Could you check a few things on this model? Use its own coordinates, in mm. Round coordinates to 2 decimals unless told otherwise and drop trailing zeros. Write each loop counter-clockwise with the first axis right and the second up, starting at its lowest first coordinate (ties: lowest second). Pieces come first, ordered by that corner, then holes. Notation, with made-up numbers: (11.25, 87) -> (31.25, 87) arc R21 cw to (31.25, 97) -> close; hole circle Ø5 at (-23, -14.75). An arc over 180 degrees is marked (long way). Return JSON: item names as keys, results as strings.
from build123d import *

# Parameters (mm, degrees)
SKETCH1_R           = 36.1315
SKETCH1_R_2         = 27.2415
BOSS_EXTRUDE1_DEPTH = 25.4
CUT_EXTRUDE1_START  = -8.908075
SKETCH2_R           = 0.9921875
CUT_EXTRUDE1_DEPTH  = 8.908075
CIRPATTERN1_COUNT   = 4


with BuildPart() as part:
    # Sketch1 → Boss-Extrude1 (new body)
    with BuildSketch(Plane(origin=(0, 0, 0), x_dir=(1, 0, 0), z_dir=(0, 1, 0))):
        Circle(SKETCH1_R)
        Circle(SKETCH1_R_2, mode=Mode.SUBTRACT)
    extrude(amount=BOSS_EXTRUDE1_DEPTH)

    # Sketch2 → Cut-Extrude1 (cut)
    with BuildSketch(Plane.XY.offset(36.1315).offset(CUT_EXTRUDE1_START)):
        with Locations((0, 12.7)):
            Circle(SKETCH2_R)
    cut_extrude1 = extrude(amount=CUT_EXTRUDE1_DEPTH, mode=Mode.SUBTRACT)

    # CirPattern1: Cut-Extrude1 ×4 about axis
    cirpattern1_axis = Axis((0, 25.4, 0), (0, -1, 0))
    for i in range(1, CIRPATTERN1_COUNT):
        add(cut_extrude1.rotate(cirpattern1_axis, i * 360 / CIRPATTERN1_COUNT), mode=Mode.SUBTRACT)


solid = part.part
1) I want a section at C-C, the plane z = 17. Please give me the cut outline in (x, y), and give its area (3 significant figures).
Return value:
{"outline": "(-31.88, 0) -> (-21.29, 0) -> (-21.29, 25.4) -> (-31.88, 25.4) -> close; (21.29, 0) -> (31.88, 0) -> (31.88, 25.4) -> (21.29, 25.4) -> close", "area": "538 mm²"}
2) I want a section at D-D, the plane y = 8.5. Please give me the cut outline in (x, z).
Return value:
{"outline": "circle Ø72.26 at (0, 0); hole circle Ø54.48 at (0, 0)"}
3) If I drill on probe 1 along Z at (x, y) = (0, 20.25); probe 2 along Y at (x, z) = (0, 33.75); probe 3 along X at (y, z) = (10.5, 8), over which ranges is the centre line in solid material (lowest first)? Write a range as [from, to].
Return value:
{"probe 1": "[-36.13, -27.24], [27.24, 36.13]", "probe 2": "[0, 11.71], [13.69, 25.4]", "probe 3": "[-35.23, -26.04], [26.04, 35.23]"}
4) I want a section at B-B, the plane z = 0. Please give me the cut outline in (x, y), and give its area (3 significant figures).
Return value:
{"outline": "(-36.13, 0) -> (-27.24, 0) -> (-27.24, 11.71) -> (-36.13, 11.71) -> close; (-36.13, 13.69) -> (-27.24, 13.69) -> (-27.24, 25.4) -> (-36.13, 25.4) -> close; (27.24, 0) -> (36.13, 0) -> (36.13, 11.71) -> (27.24, 11.71) -> close; (27.24, 13.69) -> (36.13, 13.69) -> (36.13, 25.4) -> (27.24, 25.4) -> close", "area": "416 mm²"}
5) Thinking about a two-plate mould opening in Y: for faces 1 (the face through (5, 25.4, -27)), 2 (the face through (0.215, 11.731, -31.615)), 3 (the face through (-31.615, 11.731, -0.215)), 4 (the face through (5, 0, -27)), which applies, pulls with the +Y half, pulls with the -Y half, needs draft (parallel to the pull), parting line crosses it, or undercut?
Return value:
{"face 1": "pulls with the +Y half", "face 2": "undercut", "face 3": "undercut", "face 4": "pulls with the -Y half"}
6) Will these pins go through, and if not, where does the flat tip stop? pin 1 Ø4 at (y, z) = (8, -4.5) entering from +X; pin 2 Ø6 at (y, z) = (5, 12.5) entering from -X; pin 3 Ø10 at (x, y) = (18, 5) entering from -Z.
Return value:
{"pin 1": "x = 36.04", "pin 2": "x = -34.86", "pin 3": "z = -33.71"}
7) I want a section at A-A, the plane x = 0. Please give me the cut outline in (y, z).
Return value:
{"outline": "(0, -36.13) -> (11.71, -36.13) -> (11.71, -27.24) -> (0, -27.24) -> close; (0, 27.24) -> (11.71, 27.24) -> (11.71, 36.13) -> (0, 36.13) -> close; (13.69, -36.13) -> (25.4, -36.13) -> (25.4, -27.24) -> (13.69, -27.24) -> close; (13.69, 27.24) -> (25.4, 27.24) -> (25.4, 36.13) -> (13.69, 36.13) -> close"}
